Drawing for the job (mm, zero at the part's lowest x, y, z). Round coordinates to 2 decimals unless told otherwise and drop trailing zeros. Loops run counter-clockwise (first coordinate to the right, second up) from the corner with the lowest first, then second, coordinate; pieces in that order, holes last. Notation, with made-up numbers: (44.5, 5) -> (77.5, 5) arc R15 cw to (77.5, 11) -> close; hole circle Ø11 at (-3.75, 20). An arc over 180 degrees is marked (long way). Put each result on its own line as item: value. Start each with the question number.
Item 1: Cut at C-C, the plane x = 17.5. List the corners of the cut face in (y, z).
Item 2: Flat gauge pins, fed straight in: pin 1 Ø1.2 at (x, z) = (105.5, 3) entering from +Y; pin 2 Ø1.2 at (y, z) = (59.5, 1.5) entering from +X; pin 3 Ø1.2 at (y, z) = (106, 2.5) entering from +X. Where does each tip first touch, or does it go through?
Item 3: Cut at B-B, the plane y = 75.5. List the corners of the cut face in (x, z), plus the area to 3 significant figures.
Item 4: Drill centre lines: probe 1 along X at (y, z) = (61, 0.25); probe 2 along Y at (x, z) = (64.5, 2.8); probe 3 along Y at (x, z) = (113, 3.1). Where is each one in solid material? Low to high. Write a range as [from, to].
Item 5: Cut at A-A, the plane z = 0.75. List the corners of the cut face in (x, y).
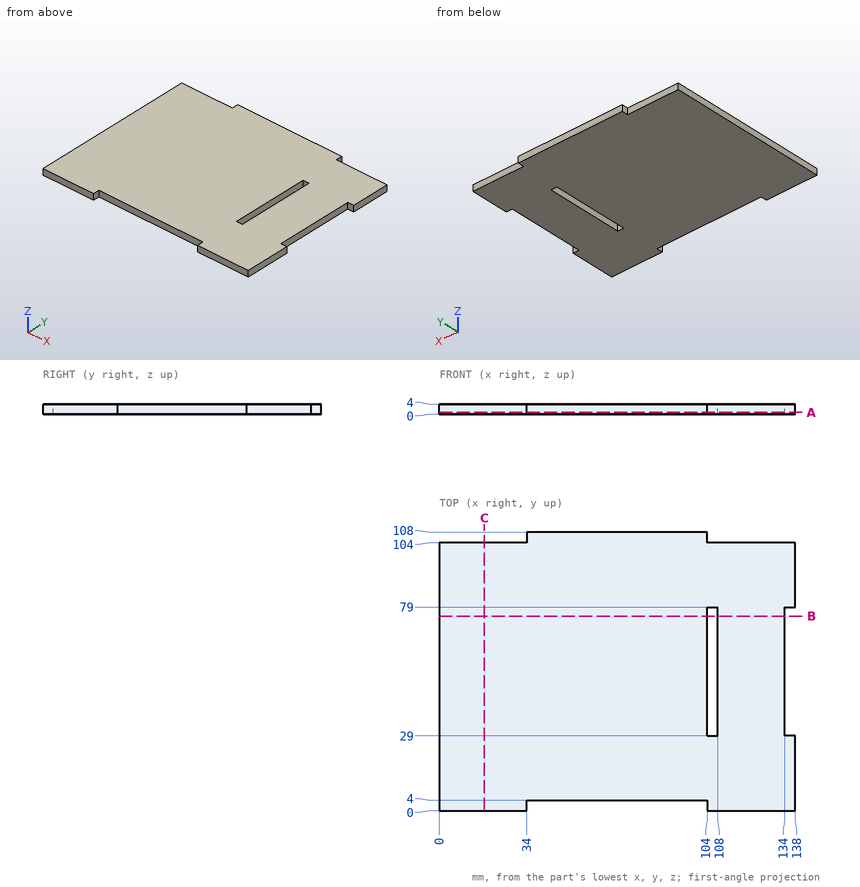
Reply:
1. outline: (0, 0) -> (104, 0) -> (104, 4) -> (0, 4) -> close
2. pin 1: stops at y = 104
2. pin 2: stops at x = 134
2. pin 3: stops at x = 104
3. outline: (0, 0) -> (104, 0) -> (104, 4) -> (0, 4) -> close; (108, 0) -> (134, 0) -> (134, 4) -> (108, 4) -> close
3. area: 520 mm^2
4. probe 1: x = [0, 104], [108, 134]
4. probe 2: y = [4, 108]
4. probe 3: y = [0, 104]
5. outline: (0, 0) -> (34, 0) -> (34, 4) -> (104, 4) -> (104, 0) -> (138, 0) -> (138, 29) -> (134, 29) -> (134, 79) -> (138, 79) -> (138, 104) -> (104, 104) -> (104, 108) -> (34, 108) -> (34, 104) -> (0, 104) -> close; hole (104, 29) -> (108, 29) -> (108, 79) -> (104, 79) -> close
